Geometry: see drawing. Coordinates: mm, zero at the bounding-box minimum. A direction names the side the tool comes from. Give positions to 0.01 mm unless a question says otherwise; leave off trailing zeros. Write each loop counter-clockwise with the first axis right and the second up, starting at its lowest first coordinate (ties: lowest second). Pieces come first, ordered by that corner, then holes. Notation, with made-up numbers: (-21, 27.5) - (30, 27.5) arc R25 cw to (30, 43.5) - close; hole circle Ø6 at (-27.75, 42). An arc over 180 degrees is marked (long way). Answer as CSV lines item,"result". Start each with the question number.
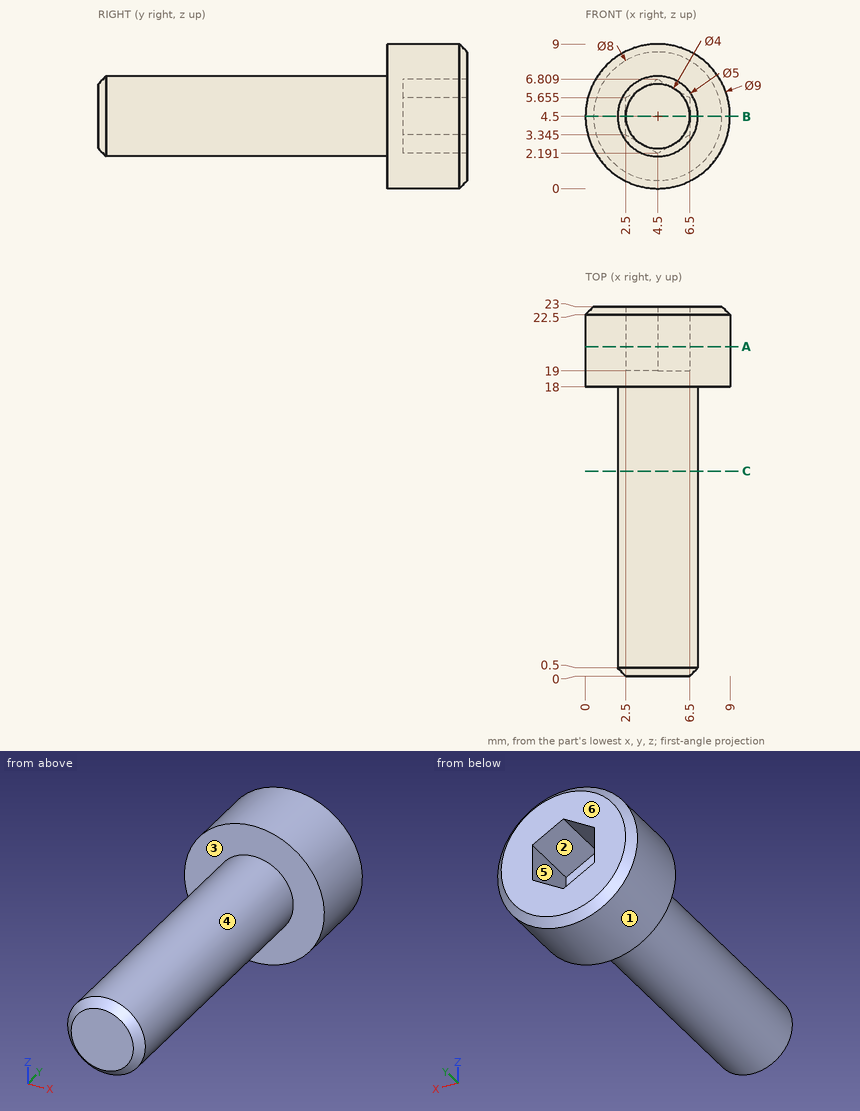
1) Cut plane A-A on y = 20.5. Output: boundary loops of the cut face in (x, z) (1 decimal).
2) Cut plane B-B on z = 4.5. Output: boundary loops of the cut face in (x, y).
3) Contact query for flat-ended pins moving along their axis: P1, Ø0.7, axis at y = 20, z = 4, coming from the -X side; P2, Ø1.5, axis at x = 2, z = 8, coming from the -Y side; P3, Ø2, axis at x = 7, y = 18, coming from the +Z side. Output: stop coordinate, or through.
4) Cut plane C-C on y = 12.75. Output: boundary loops of the cut face in (x, z).
5) Reachability of the marked faces 4, 5 and 6 from +Z, -Z, +X, -X, +Y, -Y: full face, straight path, thin tool, end or side. Return the list, or none.
6) Material intervals for line 1 (X direction, y = 5.75, z = 6); line 2 (Y direction, x = 8.25, z = 3.25); line 3 (Z direction, x = 2.75, y = 21.5) (1 decimal), sorted ascending. Write a range as from..to.
7) Pull-direction query (Z, two-part tool) for the marked faces 1, 2 and 3; classes: +Z half, -Z half, draft (parallel to the pull), parting line (faces both ways), or undercut.
Numbers:
1,outline,"circle Ø9 at (4.5, 4.5); hole (2.5, 3.3) - (4.5, 2.2) - (6.5, 3.3) - (6.5, 5.7) - (4.5, 6.8) - (2.5, 5.7) - close"
2,outline,"(0, 18) - (2, 18) - (2, 0.5) - (2.5, 0) - (6.5, 0) - (7, 0.5) - (7, 18) - (9, 18) - (9, 22.5) - (8.5, 23) - (6.5, 23) - (6.5, 19) - (2.5, 19) - (2.5, 23) - (0.5, 23) - (0, 22.5) - close"
3,P1,"stops at x = 0"
3,P2,"stops at y = 18"
3,P3,"stops at z = 8.74"
4,outline,"circle Ø5 at (4.5, 4.5)"
5,face 4,"-Y"
5,face 5,"+Y"
5,face 6,"+Z, -Z, +X, -X, +Y"
6,line 1,"x = 2.5..6.5"
6,line 2,"y = 18..23"
6,line 3,"z = 0.4..3.2, 5.8..8.6"
7,face 1,"parting line"
7,face 2,"undercut"
7,face 3,"draft"
